Check sheet for the modelled part. Datum: model origin and axes. Units: mm. Face numbers are marked on the shaded views. A direction names the side the tool comes from. Coordinates: 2 decimals unless noted, no trailing zeros. Write each loop counter-clockwise with the first axis right and the second up, starting at its lowest first coordinate (ties: lowest second). Pieces come first, ordered by that corner, then holes. Notation, with made-up numbers: M 69.25,58.25 L 102.25,58.25 A8 ccw 102.25,68.25 Z; hole C -23.5,-16.5 d2. An arc over 180 degrees is marked long. Answer as CSV lines item,"result". Start each with the question number.
1) Section check D-D (y = -3). Record the cut outline in (x, z), and give its area (3 significant figures).
2) Go/stop test with flat-tipped pins: pin 1 Ø3 at (x, z) = (1, 1) entering from +Y; pin 2 Ø1 at (y, z) = (2.5, 4.5) entering from +X; pin 3 Ø1 at (x, z) = (-2.5, 3.5) entering from -Y; pin 4 Ø0.5 at (x, z) = (-0.5, 0.5) entering from -Y. Record where each tip stops, or that it passes through.
3) Material ranges on L1, parallel to Z at x = 0.25, y = 0.25; L2, parallel to Z at x = -3, y = 1.75; L3, parallel to X at y = -0.25, z = 2.25, recorded low to high. Write a range as [from, to].
4) Draft check along Y on the marked faces 1, 2, 3 and 4. Enter one of: +Y half, -Y half, draft (parallel to the pull), parting line (faces both ways), or undercut.
5) Section check C-C (z = 2.05). Record the cut outline in (x, y), and give its area (3 significant figures).
6) Section check A-A (y = 0). Record the cut outline in (x, z).
7) Access from +Z, -Z, +X, -X, +Y, -Y to the whole of each face (thin tool, end or side, straight path). Record for the marked faces 5, 6 and 7.
from build123d import *

# Parameters (mm, degrees)
SZKIC1_R                    = 4
DODANIE_WYCI_GNI_CIE1_DEPTH = 0.75
SZKIC2_R                    = 2.9
DODANIE_WYCI_GNI_CIE2_DEPTH = 4.25
SZKIC3_W                    = 2.5
SZKIC3_H                    = 2.5
WYTNIJ_WYCI_GNI_CIE1_DEPTH  = 1
ZAOKR_GLENIE2_R             = 1
SZKIC4_W                    = 2.9
SZKIC4_H                    = 2.9
WYTNIJ_WYCI_GNI_CIE2_DEPTH  = 1


with BuildPart() as part:
    # Szkic1 → Dodanie-wyciągnięcie1 (new body)
    with BuildSketch(Plane.XY):
        Circle(SZKIC1_R)
    extrude(amount=DODANIE_WYCI_GNI_CIE1_DEPTH)

    # Szkic2 → Dodanie-wyciągnięcie2 (add)
    with BuildSketch(Plane.XY.offset(0.75)):
        Circle(SZKIC2_R)
    extrude(amount=DODANIE_WYCI_GNI_CIE2_DEPTH)

    # Szkic3 → Wytnij-wyciągnięcie1 (cut)
    with BuildSketch(Plane(origin=(0, 0, 0), x_dir=(-1, 0, 0), z_dir=(0, 0, -1))):
        Rectangle(SZKIC3_W, SZKIC3_H)
    extrude(amount=-WYTNIJ_WYCI_GNI_CIE1_DEPTH, mode=Mode.SUBTRACT)

    # Zaokrąglenie2
    zaokr_glenie2_edges = [part.edges().sort_by_distance(p)[0] for p in [
        (-2.9, 0, 5),
    ]]
    fillet(zaokr_glenie2_edges, radius=ZAOKR_GLENIE2_R)

    # Szkic4 → Wytnij-wyciągnięcie2 (cut)
    with BuildSketch(Plane(origin=(0, 0, 0), x_dir=(-1, 0, 0), z_dir=(0, 0, -1))):
        Rectangle(SZKIC4_W, SZKIC4_H)
    extrude(amount=-WYTNIJ_WYCI_GNI_CIE2_DEPTH, mode=Mode.SUBTRACT)


solid = part.part
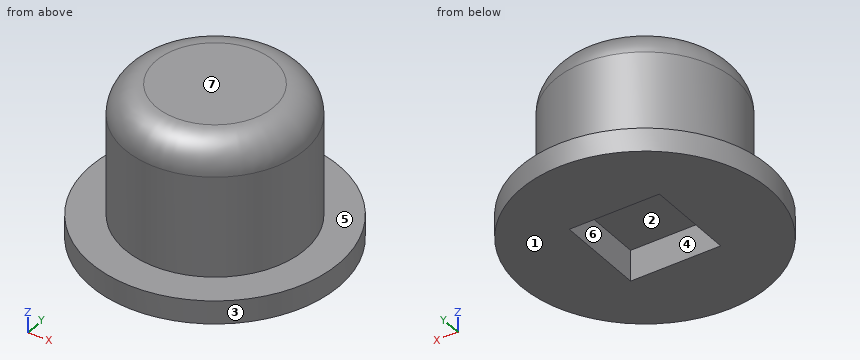
Results found:
1,outline,"M -2.65,0 L 2.65,0 L 2.65,0.75 L -2.65,0.75 Z"
1,area,"3.97 mm2"
2,pin 1,"stops at y = 4"
2,pin 2,"stops at x = 1.99"
2,pin 3,"stops at y = -2.1"
2,pin 4,"stops at y = -3.99"
3,L1,"z = [1, 5]"
3,L2,"z = [0, 0.75]"
3,L3,"x = [-2.89, 2.89]"
4,face 1,"draft"
4,face 2,"undercut"
4,face 3,"parting line"
4,face 4,"undercut"
5,outline,"C 0,0 d5.8"
5,area,"26.4 mm2"
6,outline,"M -4,0 L -1.45,0 L -1.45,1 L 1.45,1 L 1.45,0 L 4,0 L 4,0.75 L 2.9,0.75 L 2.9,4 A1 ccw 1.9,5 L -1.9,5 A1 ccw -2.9,4 L -2.9,0.75 L -4,0.75 Z"
7,face 5,"+Z"
7,face 6,"-Z"
7,face 7,"+Z, +X, -X, +Y, -Y"
